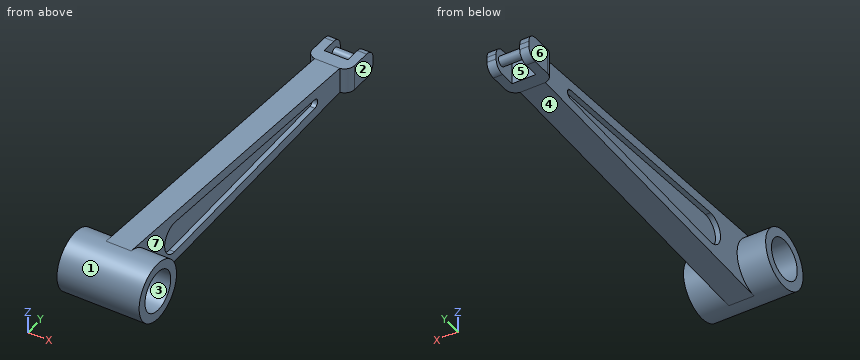
```python
from build123d import *
from build123d.topology import SkipClean

# Parameters (mm, degrees)
Y_KSEKLIK_EKSTR_ZYON2_DEPTH      = 3.75
Y_KSEKLIK_EKSTR_ZYON3_DEPTH      = 2.25
IZIM4_R                          = 6
KES_EKSTR_ZYON1_DEPTH            = 15.5
Y_KSEKLIK_EKSTR_ZYON5_DEPTH      = 8.5
Y_KSEKLIK_EKSTR_ZYON5_DEPTH_BACK = 16
IZIM5_R                          = 8.707330246
IZIM5_R_2                        = 6
IZIM1_6_W                        = 7.569576012
IZIM1_6_H                        = 4.08664072
Y_KSEKLIK_EKSTR_ZYON6_DEPTH      = 6.25
IZIM6_W                          = 2.724991533
IZIM6_H                          = 7.569576012
Y_KSEKLIK_EKSTR_ZYON7_DEPTH      = 7.5
IZIM7_R                          = 1.441213073
Y_KSEKLIK_EKSTR_ZYON8_DEPTH      = 8.5
RADYUS1_R                        = 3


with BuildPart() as part:
    # Çizim1 → Yükseklik-Ekstrüzyon2 (new, symmetric)
    with BuildSketch(Plane(origin=(0, 0, 0), x_dir=(0, 0, -1), z_dir=(1, 0, 0))):
        with BuildLine():
            Line((3.784788006, 102.00780299), (-3.784788006, 102.00780299))
            Line((-3.784788006, 102.00780299), (-8.707330246, 4.05112335))
            ThreePointArc((-8.707330246, 4.05112335), (0, -4.656206896), (8.707330246, 4.05112335))
            Line((8.707330246, 4.05112335), (3.784788006, 102.00780299))
        make_face()
        with BuildLine():
            Line((-4.643687916, 25.141862002), (-1.364548141, 90.395470555))
            ThreePointArc((-1.364548141, 90.395470555), (0, 91.693168951), (1.364548141, 90.395470555))
            Line((1.364548141, 90.395470555), (4.643687916, 25.141862002))
            ThreePointArc((4.643687916, 25.141862002), (0, 20.498174086), (-4.643687916, 25.141862002))
        make_face(mode=Mode.SUBTRACT)
    extrude(amount=Y_KSEKLIK_EKSTR_ZYON2_DEPTH, both=True)

    # Çizim1<5> → Yükseklik-Ekstrüzyon3 (add, symmetric)
    with BuildSketch(Plane(origin=(0, 0, 0), x_dir=(0, 0, -1), z_dir=(1, 0, 0))):
        with BuildLine():
            Line((-1.364548141, 90.395470555), (-4.643687916, 25.141862002))
            ThreePointArc((-4.643687916, 25.141862002), (0, 20.498174086), (4.643687916, 25.141862002))
            Line((4.643687916, 25.141862002), (1.364548141, 90.395470555))
            ThreePointArc((1.364548141, 90.395470555), (0, 91.693168951), (-1.364548141, 90.395470555))
        make_face()
    extrude(amount=Y_KSEKLIK_EKSTR_ZYON3_DEPTH, both=True)

    # Çizim4 → Kes-Ekstrüzyon1 (cut)
    with BuildSketch(Plane(origin=(3.75, 0, 0), x_dir=(0, 0, -1), z_dir=(1, 0, 0))):
        with Locations((0, 4.05112335)):
            Circle(IZIM4_R)
    extrude(amount=-KES_EKSTR_ZYON1_DEPTH, mode=Mode.SUBTRACT)

    # Çizim5 → Yükseklik-Ekstrüzyon5 (add, two sides: drawn at the far end of the back side and taken through both)
    with SkipClean():  # the faces are left unmerged after this step: merging them gives an invalid solid
        with BuildSketch(Plane(origin=(3.75, 0, 0), x_dir=(0, 0, -1), z_dir=(1, 0, 0)).offset(-Y_KSEKLIK_EKSTR_ZYON5_DEPTH_BACK)):
            with Locations((0, 4.05112335)):
                Circle(IZIM5_R)
            with Locations((0, 4.05112335)):
                Circle(IZIM5_R_2, mode=Mode.SUBTRACT)
        extrude(amount=Y_KSEKLIK_EKSTR_ZYON5_DEPTH + Y_KSEKLIK_EKSTR_ZYON5_DEPTH_BACK)

    # Çizim1<6> → Yükseklik-Ekstrüzyon6 (add, symmetric)
    with BuildSketch(Plane(origin=(0, 0, 0), x_dir=(0, 0, -1), z_dir=(1, 0, 0))):
        with Locations((0, 104.05112335)):
            Rectangle(IZIM1_6_W, IZIM1_6_H)
    extrude(amount=Y_KSEKLIK_EKSTR_ZYON6_DEPTH, both=True)

    # Çizim6 → Yükseklik-Ekstrüzyon7 (add)
    with BuildSketch(Plane(origin=(0, 106.09444371, 0), x_dir=(1, 0, 0), z_dir=(0, 1, 0))):
        with Locations((-4.887504233, 0)):
            Rectangle(IZIM6_W, IZIM6_H)
        with Locations((4.887504233, 0)):
            Rectangle(IZIM6_W, IZIM6_H)
    extrude(amount=Y_KSEKLIK_EKSTR_ZYON7_DEPTH)

    # Çizim7 → Yükseklik-Ekstrüzyon8 (add)
    with BuildSketch(Plane(origin=(-3.525008467, 0, 0), x_dir=(0, 0, -1), z_dir=(1, 0, 0))):
        with Locations(Location((0, 111.076861872, 0), (0, 0, 180))):
            Circle(IZIM7_R)
    extrude(amount=Y_KSEKLIK_EKSTR_ZYON8_DEPTH)

    # Radyus1
    # the kernel refuses this fillet: 3 mm, written as the material it takes off along each edge
    with BuildSketch(Plane(origin=(6.25, 102.00780299, -11.179887735), x_dir=(0, 1, 0), z_dir=(0, 0, 1))) as radyus1_piece_1:
        with BuildLine():
            CenterArc((2.958039892, 3), RADYUS1_R, 189.594068227, 80.405931773)
            Line((0, 2.5), (-0.059160798, 2.49))
            ThreePointArc((-0.059160798, 2.49), (-0.06, 1.25), (-0.06, 0))
            Line((-0.06, 0), (0, -0.06))
            Line((0, -0.06), (2.958039892, -0.06))
            Line((2.958039892, -0.06), (2.958039892, 0))
        make_face()
    extrude(amount=22.359775471, mode=Mode.SUBTRACT)
    with BuildSketch(Plane(origin=(-6.25, 102.00780299, -11.179887735), x_dir=(1, 0, 0), z_dir=(0, 0, 1))) as radyus1_piece_2:
        with BuildLine():
            CenterArc((3, 2.958039892), RADYUS1_R, 180, 80.405931773)
            Line((0, 2.958039892), (-0.06, 2.958039892))
            Line((-0.06, 2.958039892), (-0.06, 0))
            Line((-0.06, 0), (0, -0.06))
            ThreePointArc((0, -0.06), (1.25, -0.06), (2.49, -0.059160798))
            Line((2.49, -0.059160798), (2.5, 0))
        make_face()
    extrude(amount=22.359775471, mode=Mode.SUBTRACT)
    with BuildSketch(Plane(origin=(13.75, 113.59444371, 3.784788006), x_dir=(0, -1, 0), z_dir=(-1, 0, 0)), Plane(origin=(-3.974991533, 113.59444371, -3.784788006), x_dir=(0, -1, 0), z_dir=(1, 0, 0)), Plane(origin=(-13.75, 113.59444371, -3.784788006), x_dir=(0, -1, 0), z_dir=(1, 0, 0)), Plane(origin=(3.974991533, 113.59444371, 3.784788006), x_dir=(0, -1, 0), z_dir=(-1, 0, 0))) as radyus1_piece_3:
        with BuildLine():
            CenterArc((RADYUS1_R, -RADYUS1_R), RADYUS1_R, 90, 90)
            Line((0, -RADYUS1_R), (-RADYUS1_R * 0.02, -RADYUS1_R))
            Line((-RADYUS1_R * 0.02, -RADYUS1_R), (-RADYUS1_R * 0.02, RADYUS1_R * 0.02))
            Line((-RADYUS1_R * 0.02, RADYUS1_R * 0.02), (RADYUS1_R, RADYUS1_R * 0.02))
            Line((RADYUS1_R, RADYUS1_R * 0.02), (RADYUS1_R, 0))
        make_face()
    extrude(amount=17.724991533, mode=Mode.SUBTRACT)


solid = part.part
```
Part model, mm, in its own coordinate system. Face numbers are marked on the shaded views. A direction names the side the tool comes from. Coordinates: 2 decimals unless noted, no trailing zeros. Order: outer loops, then holes, each group sorted by start corner. A loop starts at its lowest first (then second) coordinate and runs counter-clockwise, first axis right, second up. Notation, with made-up numbers: (-27, -30.5) - (12, -30.5) arc R23 cw to (12, -11.5) - close; hole circle Ø6 at (3, 45.5). An arc over 180 degrees is marked (long way). Return JSON: item names as keys, results as strings. Group by question number.
Item 1: Which spindle directions (+Z, -Z, +X, -X, +Y, -Y) get a long thin tool onto all of the face, cutting with end or side? Do the marked faces 1, 2 and 3. Say none if no direction does.
Item 2: Cut at D-D (y = 42.5). List the corners of the cut face in (x, z).
Item 3: Pin check, flat tips, straight feed: pin 1 (10 mm diameter, centred on y = 62.5, z = 2, fed in from -X); pin 2 (6 mm diameter, centred on y = 109, z = -1.5, fed in from +X); pin 3 (5.5 mm diameter, centred on x = -1.5, z = -1, fed in from +Y); pin 4 (2 mm diameter, centred on y = 111.5, z = 1.5, fed in from +X). Stop position of each tip, or through.
Item 4: Cut at A-A (x = -0.75). List the corners of the cut face in (y, z).
Item 5: Drill centre lines: probe 1 along Y at (x, z) = (-1.5, 0); probe 2 along Y at (x, z) = (-2.75, 0); probe 3 along Y at (x, z) = (6.75, 0). Where is each one in solid material? Low to high. Write a range as from..to.
Item 6: Cut at B-B (y = 80.5). List the corners of the cut face in (x, z).
Item 7: Cut at C-C (x = 7.75). List the corners of the cut face in (y, z), plus the area to 3 significant figures.
Item 8: Pull direction X, two halves, no side cores. Call the marked faces 4, 5, 6 and 7: pulls with the +X half, pulls with the -X half, needs draft (parallel to the pull), parting line crosses it, or undercut.
Check values:
{
 "1": {"face 1": "none", "face 2": "+Z, -Z, +X, +Y", "face 3": "+X, -X"},
 "2": {"outline": "(-3.75, -6.78) - (3.75, -6.78) - (3.75, -3.77) - (2.25, -3.77) - (2.25, 3.77) - (3.75, 3.77) - (3.75, 6.78) - (-3.75, 6.78) - (-3.75, 3.77) - (-2.25, 3.77) - (-2.25, -3.77) - (-3.75, -3.77) - close"},
 "3": {"pin 1": "stops at x = -3.75", "pin 2": "stops at x = 6.25", "pin 3": "stops at y = 113.59", "pin 4": "stops at x = 6.25"},
 "4": {"outline": "(4.92, -8.66) - (102.01, -3.78) - (106.09, -3.78) - (106.09, 3.78) - (102.01, 3.78) - (4.92, 8.66) arc R8.71 ccw (long way) to start; circle Ø2.88 at (111.08, 0); hole circle Ø12 at (4.05, 0)"},
 "5": {"probe 1": "y = -4.66..-1.95, 10.05..106.09, 109.64..112.52", "probe 2": "y = -4.66..-1.95, 10.05..20.5, 91.69..106.09, 109.64..112.52", "probe 3": "y = -4.66..-1.95, 10.05..12.76"},
 "6": {"outline": "(-3.75, -4.87) - (3.75, -4.87) - (3.75, -1.86) - (2.25, -1.86) - (2.25, 1.86) - (3.75, 1.86) - (3.75, 4.87) - (-3.75, 4.87) - (-3.75, 1.86) - (-2.25, 1.86) - (-2.25, -1.86) - (-3.75, -1.86) - close"},
 "7": {"outline": "circle Ø17.41 at (4.05, 0); hole circle Ø12 at (4.05, 0)", "area": "125 mm2"},
 "8": {"face 4": "needs draft", "face 5": "undercut", "face 6": "pulls with the -X half", "face 7": "pulls with the +X half"}
}
